For this review, take the finished solid that the model builds, in its own axes (mm). A direction names the side the tool comes from. Round coordinates to 2 decimals unless told otherwise and drop trailing zeros. Loops run counter-clockwise (first coordinate to the right, second up) from the corner with the lowest first, then second, coordinate; pieces in that order, holes last.
1) Take a section at B-B (y = -4.1). State the section outline as (x, z) points.
2) Wall thickness on L1, parallel to Z at x = -23.5, y = -4.25; L2, parallel to X at y = -0.75, z = -78; L3, parallel to Z at x = -22, y = -3.65: over which ranges is each line inside the solid? List them lowest first.
3) Take a section at A-A (x = 0). State the section outline as (y, z) points, then the cut area to 3 significant figures.
4) Mouldability with a two-part tool opening along X and no side actions: class faces 1 (the flat face through (-8, -5, -40)), 2 (the cylindrical face through (-0.791, -2.465, 21.466)), 3 (the cylindrical face through (-27.201, -2.465, -87.427)), 4 (the flat face through (12.19, -2.465, -70.255)) as pulls with the +X half, pulls with the -X half, needs draft (parallel to the pull), parting line crosses it, or undercut.
5) Take a section at D-D (x = 15.5). State the section outline as (y, z) points, then the cut area to 3 significant figures.
6) Tool access review of faces 5 (the flat face through (-8.9, -2.5, -75)), 6 (the flat face through (-8, 0, -40)): name each direction out of +Z, -Z, +X, -X, +Y, -Y from which nothing blocks a thin tool from reaching the whole face with its end or side.
7) Take a section at C-C (z = 17.5). State the section outline as (x, y) points, then the cut area to 3 significant figures.
8) Insertion check: pin 1 (4.5 mm diameter, centred on x = 0, z = 25.03, fed in from +Y); pin 2 (3 mm diameter, centred on y = -3.5, z = -5.5, fed in from +X); pin 3 (1 mm diameter, centred on y = -2.5, z = -66, fed in from -X). Each pin has a flat end and moves straight along its axis. Give the tip position at first contact, or say it passes through.
```python
from build123d import *

# Parameters (mm, degrees)
F0_R     = 3.65
F1_DEPTH = 5


with BuildPart() as f1:
    # F0 (on Front) → F1 (new body)
    with BuildSketch(Plane.XZ):
        with BuildLine():
            Line((18.738222, -26.13953), (8.994647, 25.339406))
            ThreePointArc((8.994647, 25.339406), (0.659117, 34.004884), (-8.852828, 26.649989))
            ThreePointArc((-8.852828, 26.649989), (-9.264911, 25.107257), (-9.9173, 23.649785))
            Line((-9.9173, 23.649785), (-22.407404, 0.830026))
            ThreePointArc((-22.407404, 0.830026), (-24.572798, -1.875574), (-27.531595, -3.679662))
            ThreePointArc((-27.531595, -3.679662), (-48.884356, -28.469314), (-40.421234, -60.073789))
            ThreePointArc((-40.421234, -60.073789), (-39.132184, -61.805731), (-38.244918, -63.773987))
            Line((-38.244918, -63.773987), (-34.476732, -75.324515))
            ThreePointArc((-34.476732, -75.324515), (-34.096429, -76.928149), (-33.984688, -78.572467))
            ThreePointArc((-33.984688, -78.572467), (-27.035203, -87.467818), (-16.861534, -82.577107))
            ThreePointArc((-16.861534, -82.577107), (-15.643593, -80.633495), (-14.014829, -79.018525))
            Line((-14.014829, -79.018525), (-3.553493, -70.79486))
            ThreePointArc((-3.553493, -70.79486), (0.233142, -68.947223), (4.444673, -68.823224))
            Line((4.444673, -68.823224), (20.155766, -71.728023))
            ThreePointArc((20.155766, -71.728023), (21.115911, -71.955038), (22.049012, -72.275563))
            ThreePointArc((22.049012, -72.275563), (33.646241, -67.499015), (29.20736, -55.768394))
            Line((29.20736, -55.768394), (22.479737, -48.278609))
            ThreePointArc((22.479737, -48.278609), (20.385469, -44.614186), (19.989534, -40.412139))
            ThreePointArc((19.989534, -40.412139), (20.102008, -33.211121), (18.738222, -26.13953))
        make_face()
        with Locations((-24.985654, -78.704294)):
            Circle(F0_R, mode=Mode.SUBTRACT)
        with Locations((25.389197, -63.918341)):
            Circle(F0_R, mode=Mode.SUBTRACT)
        with Locations((0, 25.029052)):
            Circle(F0_R, mode=Mode.SUBTRACT)
    extrude(amount=F1_DEPTH)


solid = f1.part
```
Response:
1. outline: (-40.42, -60.07) arc R10 cw to (-38.24, -63.77) - (-34.48, -75.32) arc R10 cw to (-33.98, -78.57) arc R9 ccw to (-16.86, -82.58) arc R10 cw to (-14.01, -79.02) - (-3.55, -70.79) arc R10 cw to (4.44, -68.82) - (20.16, -71.73) arc R10 cw to (22.05, -72.28) arc R9 ccw to (29.21, -55.77) - (22.48, -48.28) arc R10 cw to (19.99, -40.41) arc R35 ccw to (18.74, -26.14) - (8.99, 25.34) arc R9 ccw to (-8.85, 26.65) arc R10 cw to (-9.92, 23.65) - (-22.41, 0.83) arc R10 cw to (-27.53, -3.68) arc R35 ccw to start; hole circle Ø7.3 at (-24.99, -78.7); hole circle Ø7.3 at (0, 25.03); hole circle Ø7.3 at (25.39, -63.92)
2. L1: z = -87.58 to -82.04, -75.37 to -0.77
2. L2: x = -33.99 to -28.57, -21.4 to -12.72
2. L3: z = -87.19 to -80.8, -76.6 to 1.57
3. outline: (-5, -69.01) - (0, -69.01) - (0, 21.38) - (-5, 21.38) - close; (-5, 28.68) - (0, 28.68) - (0, 34.03) - (-5, 34.03) - close
3. area: 479 mm2
4. face 1: needs draft
4. face 2: undercut
4. face 3: parting line crosses it
4. face 4: undercut
5. outline: (-5, -70.87) - (0, -70.87) - (0, -9.03) - (-5, -9.03) - close
5. area: 309 mm2
6. face 5: -Z, +Y, -Y
6. face 6: +Z, -Z, +X, -X, +Y
7. outline: (-13.28, -5) - (10.48, -5) - (10.48, 0) - (-13.28, 0) - close
7. area: 119 mm2
8. pin 1: passes through
8. pin 2: stops at x = 15.12
8. pin 3: stops at x = -37.68
